Work out the finished part from the listing and answer in its coordinate system (mm). A direction names the side the tool comes from. Round coordinates to 2 decimals unless told otherwise and drop trailing zeros. Order: outer loops, then holes, each group sorted by start corner. A loop starts at its lowest first (then second) coordinate and runs counter-clockwise, first axis right, second up. Notation, with made-up numbers: M -10,-15.5 L 36,-15.5 A20 ccw 36,-10.5 Z; hole C 66.25,-7.5 d5. An arc over 180 degrees is marked long. Return JSON: item names as keys, results as strings.
Autodesk Inventor part; units mm, degrees
ref_plane "YZ Plane" through (0, 0, 0) normal (1, 0, 0) x (0, 1, 0)
ref_plane "XZ Plane" through (0, 0, 0) normal (0, 1, 0) x (-1, 0, 0)
ref_plane "XY Plane" through (0, 0, 0) normal (0, 0, 1) x (1, 0, 0)
sketch "Эскиз1" plane through (0, 0, 0) normal (0, 0, 1) x (1, 0, 0)
  line L0 (50, -75) -> (-50, -75)
  line L1 (-50, -75) -> (-50, 75)
  line L2 (-50, 75) -> (50, 75)
  line L3 (50, 75) -> (50, -75)
  line L4 (50, -75) -> (-50, 75) construction
  line L5 (-50, -75) -> (50, 75) construction
  point P0 (0, 0)
  dimension "d0" = 100
  dimension "d1" = 150
extrude "Выдавливание1" add sketch "Эскиз1" along normal blind 3
sketch "Эскиз2" plane through (0, 0, 3) normal (0, 0, 1) x (1, 0, 0)
  line L0 (-50, 75) -> (-50, -75)
  line L1 (50, -75) -> (-50, -75)
  line L2 (-50, -75) -> (-50, 75)
  line L3 (-50, 75) -> (50, 75)
  line L4 (50, 75) -> (50, -75)
  line L5 (50, -75) -> (-50, 75) construction
  line L6 (-50, -75) -> (50, 75) construction
  line L7 (-50.1414, 75) -> (-50.1414, -75)
  line L8 (40, 65) -> (-40, 65)
  line L9 (-40, 65) -> (-40, -65)
  line L10 (-40, -65) -> (40, -65)
  line L11 (40, -65) -> (40, 65)
  point P0 (0, 0)
  dimension "d4" = 10
extrude "Выдавливание2" add sketch "Эскиз2" along normal blind 10
sketch "Эскиз3" plane through (0, 0, 0) normal (1, 0, 0) x (0, 1, 0)
  line L0 (0, 0) -> (-75, -20.0962)
  line L1 (-75, 0) -> (75, 0)
  line L2 (-75, -20.0962) -> (-75, 0)
  line L3 (-75, 0) -> (0, 0)
  dimension "d7" = 15
extrude "Выдавливание3" add sketch "Эскиз3" along normal mid plane 20
properties part number "project2"
Item 1: Find section C-C (y = 15). Determine the outline of the cut face in (x, z), plus the area to 3 significant figures.
Output:
{"outline": "M -50,0 L 50,0 L 50,13 L 40,13 L 40,3 L -40,3 L -40,13 L -50,13 Z", "area": "500 mm^2"}
Item 2: Find section A-A (z = 10.5). Determine the outline of the cut face in (x, y).
Output:
{"outline": "M -50,-75 L 50,-75 L 50,75 L -50,75 Z; hole M -40,-65 L 40,-65 L 40,65 L -40,65 Z"}
Item 3: Find section B-B (x = -6). Determine the outline of the cut face in (y, z), plus the area to 3 significant figures.
Output:
{"outline": "M -75,-20.1 L 0,0 L 75,0 L 75,13 L 65,13 L 65,3 L -65,3 L -65,13 L -75,13 Z", "area": "1,400 mm^2"}
Item 4: Consider line 1 along X through (y, z) = (9.5, 3.5); line 2 along Z through (x, y) = (-38, 0.5); line 3 along X through (y, z) = (-67.5, -4.5). Determine where each line is inside the solid, lowest interval first. Write a range as [from, to].
Output:
{"line 1": "x = [-50, -40], [40, 50]", "line 2": "z = [0, 3]", "line 3": "x = [-10, 10]"}
Item 5: Which of the six approach directions +Z, -Z, +X, -X, +Y, -Y give full straight-line access (tool end or side, diameter ignored) to faces 4 (the flat face through (1, 65, 8)), 5 (the flat face through (-1, 75, 6)), 6 (the flat face through (-10, -46, -8))?
Output:
{"face 4": "+Z", "face 5": "+Z, -Z, +X, -X, +Y", "face 6": "-Z, -X, +Y, -Y"}
Item 6: The mould has two halves that part along X. Classify faces 1 (the flat face through (-45, 1, 13)), 2 (the flat face through (10, -46, -8)), 3 (the flat face through (-40, 1, 8)): pulls with the +X half, pulls with the -X half, needs draft (parallel to the pull), parting line crosses it, or undercut.
Output:
{"face 1": "needs draft", "face 2": "pulls with the +X half", "face 3": "undercut"}
Item 7: Find section D-D (x = -24.5). Determine the outline of the cut face in (y, z), plus the area to 3 significant figures.
Output:
{"outline": "M -75,0 L 75,0 L 75,13 L 65,13 L 65,3 L -65,3 L -65,13 L -75,13 Z", "area": "650 mm^2"}
Item 8: Each of these flat-tipped pins is pushed along its axis until it touches: pin 1 (1.5 mm diameter, centred on x = 31.5, y = 55.5, fed in from +Z); pin 2 (12 mm diameter, centred on x = 12.5, y = 52.5, fed in from -Z). Where does it stop, or does it pass through?
Output:
{"pin 1": "stops at z = 3", "pin 2": "stops at z = 0"}
